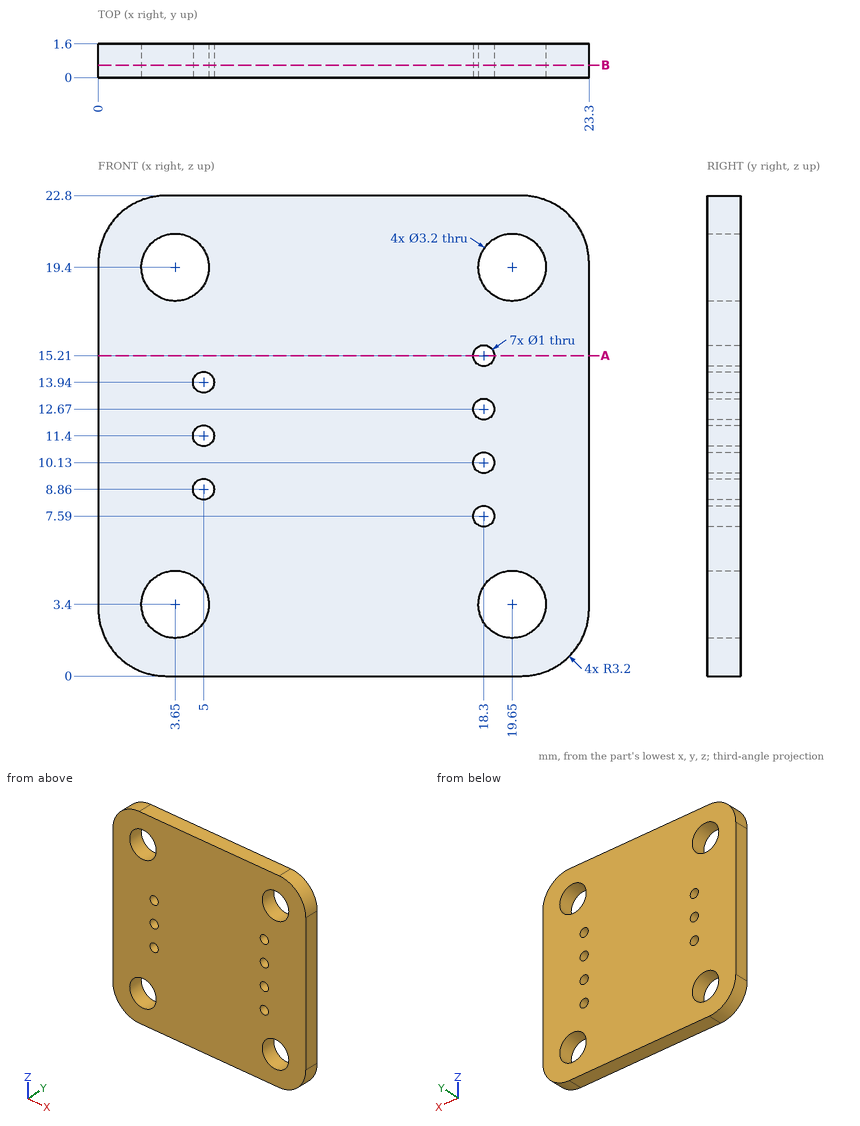
The figure shows three views and two pictorial views of one solid part (mm, origin at its lowest corner). Answer the questions. Give positions to 0.01 mm unless a question says otherwise; leave off trailing zeros. Write each loop counter-clockwise with the first axis right and the second up, starting at its lowest first coordinate (ties: lowest second). Pieces come first, ordered by that corner, then holes. Notation, with made-up numbers: (56, 43) - (80, 43) arc R35 ccw to (80, 76) - close; hole circle Ø6 at (45, 46.25). An arc over 180 degrees is marked (long way). Use CSV: the item, a comma, the result in double quotes. Start each with the question number.
Item 1: The part is cut by section A-A, the plane z = 15.21. Give the vertices of the cut face in (x, y).
Item 2: Consider line 1 (X direction, y = 0.9, z = 3.4); line 2 (X direction, y = 0.7, z = 12.67); line 3 (X direction, y = 0.4, z = 14). Determine where each line is inside the solid, lowest interval first.
Item 3: The part is cut by section B-B, the plane y = 0.6. Count the separate pieces of the cut face and the enclosed holes in it, and give its area (3 significant figures).
Taken from the geometry:
1,outline,"(0, 0) - (17.8, 0) - (17.8, 1.6) - (0, 1.6) - close; (18.8, 0) - (23.3, 0) - (23.3, 1.6) - (18.8, 1.6) - close"
2,line 1,"0 to 2.05, 5.25 to 18.05, 21.25 to 23.3"
2,line 2,"0 to 17.8, 18.8 to 23.3"
2,line 3,"0 to 4.5, 5.5 to 23.3"
3,separate pieces,"1"
3,enclosed holes,"11"
3,area,"485 mm2"
